Verification items for the finished model (mm, model axes). Face numbers are marked on the shaded views. A direction names the side the tool comes from. Round coordinates to 2 decimals unless told otherwise and drop trailing zeros. Order: outer loops, then holes, each group sorted by start corner. A loop starts at its lowest first (then second) coordinate and runs counter-clockwise, first axis right, second up. Notation, with made-up numbers: M 49.5,54.25 L 54.5,54.25 A19 cw 54.5,66.25 Z; hole C 43,69.25 d9. An arc over 180 degrees is marked long. Use CSV: the item, a comma, the result in double quotes. Start each with the question number.
Q1. Scan lines: line 1 (Z direction, x = 3.81, y = -4.7); line 2 (Y direction, x = 3, z = -6.5); line 3 (Y direction, x = 2.25, z = -15) (3 decimals). Record each from-to range of solid material in increasing order.
Q2. Sectioned sample at D-D (y = -91). Enter the section's corners in (x, z), and give its area (3 significant figures).
Q3. Sectioned sample at B-B (z = -4.5). Enter the section's corners in (x, y) (3 decimals).
Q4. Gauge pin test, flat ends, axial feed: pin 1 Ø4.5 at (x, y) = (8.26, -77.05) entering from -Z; pin 2 Ø1.7 at (x, y) = (9.5, -86) entering from +Z; pin 3 Ø4.5 at (x, z) = (3.81, -13.97) entering from -Y (3 decimals); pin 4 Ø3 at (x, z) = (3.81, -21.59) entering from -Y. Record the tip position at first contact, or that the pin passes through.
Q5. Sectioned sample at A-A (x = 3.81). Enter the section's corners in (y, z) (3 decimals), and give its area (3 significant figures).
Q6. Sectioned sample at C-C (z = -13.97). Enter the section's corners in (x, y) (3 decimals), and give its area (3 significant figures).
Q7. Set-up check for the marked faces 1, 2, 3 and 4: record each of +Z, -Z, +X, -X, +Y, -Y from which the full face is reachable in a straight line by a thin tool's end or side.
Q8. Mould release check, pull along Y, two halves, no side actions. Record for the marked faces 5, 6 and 7: +Y half, -Y half, draft (parallel to the pull), parting line (faces both ways), or undercut.
```python
from build123d import *

# Parameters (mm, degrees)
SKETCH1_W                                      = 12.7
SKETCH1_H                                      = 96.5962
EXTRUDE1_DEPTH                                 = 5.08
SKETCH2_W                                      = 12.7
SKETCH2_H                                      = 5.16498089
EXTRUDE2_DEPTH                                 = 25.4
F_4_CLEARANCE_HOLE1_D                          = 3.4544
SKETCH6_W                                      = 12.7
SKETCH6_H                                      = 22.86
EXTRUDE4_DEPTH                                 = 7.62
SKETCH7_W                                      = 7.9248
SKETCH7_H                                      = 15.24
EXTRUDE5_DEPTH                                 = 3.175
FILLET1_R                                      = 1.27
FILLET3_R                                      = 6.35
CHAMFER1_SIZE                                  = 0.762
CBORE_FOR_4_SOCKET_HEAD_CAP_SCREW1_D           = 3.4544
CBORE_FOR_4_SOCKET_HEAD_CAP_SCREW1_CBORE_D     = 5.55752
CBORE_FOR_4_SOCKET_HEAD_CAP_SCREW1_CBORE_DEPTH = 2.8448


with BuildPart() as part:
    # Sketch1 → Extrude1 (new body)
    with BuildSketch(Plane.XY):
        with Locations((6.35, -48.2981)):
            Rectangle(SKETCH1_W, SKETCH1_H)
    extrude(amount=EXTRUDE1_DEPTH)

    # Sketch2 → Extrude2 (add)
    with BuildSketch(Plane(origin=(0, 0, 0), x_dir=(-1, 0, 0), z_dir=(0, 0, -1))):
        with Locations((-6.35, -2.582490445)):
            Rectangle(SKETCH2_W, SKETCH2_H)
    extrude(amount=EXTRUDE2_DEPTH)

    # #4 Clearance Hole1 (through all)
    with Locations(Plane(origin=(0, 0, 0), x_dir=(-1, 0, 0), z_dir=(0, 1, 0))):
        with Locations((-3.81, -21.59), (-3.81, -13.97)):
            Hole(F_4_CLEARANCE_HOLE1_D / 2)

    # Sketch6 → Extrude4 (add)
    with BuildSketch(Plane(origin=(0, 0, 0), x_dir=(-1, 0, 0), z_dir=(0, 0, -1))):
        with Locations((-6.35, -85.1662)):
            Rectangle(SKETCH6_W, SKETCH6_H)
    extrude(amount=EXTRUDE4_DEPTH)

    # Sketch7 → Extrude5 (cut)
    with BuildSketch(Plane(origin=(0, 0, 0), x_dir=(1, 0, 0), z_dir=(0, 1, 0))):
        with Locations((3.81, 17.78)):
            Rectangle(SKETCH7_W, SKETCH7_H)
    extrude(amount=-EXTRUDE5_DEPTH, mode=Mode.SUBTRACT)

    # Fillet1
    fillet1_edges = [part.edges().sort_by_distance(p)[0] for p in [
        (7.7724, -1.5875, -10.16),
    ]]
    fillet(fillet1_edges, radius=FILLET1_R)

    # Fillet3
    fillet3_edges = [part.edges().sort_by_distance(p)[0] for p in [
        (6.35, -5.16498089, 0),
        (6.35, -73.7362, 0),
    ]]
    fillet(fillet3_edges, radius=FILLET3_R)

    # Chamfer1
    chamfer1_edges = [part.edges().sort_by_distance(p)[0] for p in [
        (12.7, -48.2981, 5.08),
        (6.35, 0, 5.08),
        (0, -48.2981, 5.08),
        (6.35, -96.5962, 5.08),
    ]]
    chamfer(chamfer1_edges, length=CHAMFER1_SIZE)

    # CBORE for #4 Socket Head Cap Screw1 (through all)
    with Locations(Plane.XY.offset(5.08)):
        with Locations((8.255, -84.97178089), (8.255, -77.04698089)):
            CounterBoreHole(CBORE_FOR_4_SOCKET_HEAD_CAP_SCREW1_D / 2, CBORE_FOR_4_SOCKET_HEAD_CAP_SCREW1_CBORE_D / 2, CBORE_FOR_4_SOCKET_HEAD_CAP_SCREW1_CBORE_DEPTH)


solid = part.part
```
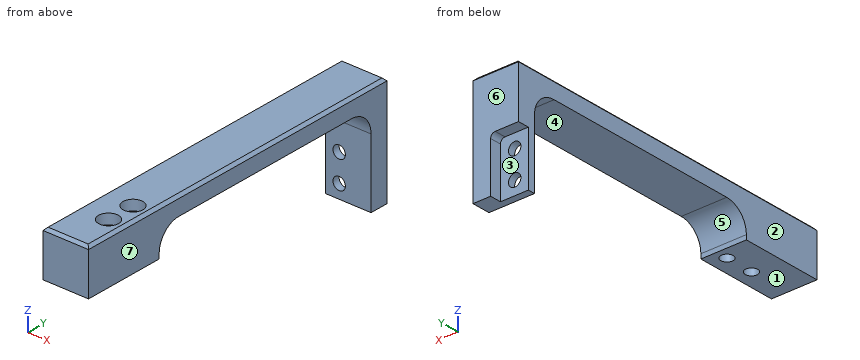
Verdict:
1,line 1,"z = -25.4 to -23.32, -19.86 to -15.7, -12.24 to 5.08"
1,line 2,"y = -96.6 to -73.74, -5.16 to 0"
1,line 3,"y = -5.165 to -3.175"
2,outline,"M 0,-7.62 L 12.7,-7.62 L 12.7,4.32 L 11.94,5.08 L 0.76,5.08 L 0,4.32 Z"
2,area,"161 mm²"
3,outline,"M 0,-96.596 L 12.7,-96.596 L 12.7,-73.461 L 0,-73.461 Z; M 0,-5.44 L 12.7,-5.44 L 12.7,0 L 0,0 Z; hole C 8.255,-84.972 d3.454; hole C 8.255,-77.047 d3.454"
4,pin 1,"stops at z = -7.62"
4,pin 2,"stops at z = 2.24"
4,pin 3,"stops at y = -5.165"
4,pin 4,"passes through"
5,outline,"M -96.596,-7.62 L -73.736,-7.62 L -73.736,-6.35 A6.35 cw -67.386,0 L -11.515,0 A6.35 cw -5.165,-6.35 L -5.165,-12.243 L -3.175,-12.243 L -3.175,-10.16 L 0,-10.16 L 0,4.318 L -0.762,5.08 L -95.834,5.08 L -96.596,4.318 Z; M -5.165,-25.4 L -3.175,-25.4 L -3.175,-23.317 L -5.165,-23.317 Z; M -5.165,-19.863 L -3.175,-19.863 L -3.175,-15.697 L -5.165,-15.697 Z"
5,area,"751 mm²"
6,outline,"M 0,-5.165 L 2.083,-5.165 L 2.083,-3.175 L 0,-3.175 Z; M 5.537,-5.165 L 12.7,-5.165 L 12.7,0 L 7.772,0 L 7.772,-3.175 L 5.537,-3.175 Z"
6,area,"34.0 mm²"
7,face 1,"-Z, +X, -X, -Y"
7,face 2,"+Z, -Z, -X, +Y, -Y"
7,face 3,"-Z, -X, +Y"
7,face 4,"-Z, +X, -X"
8,face 5,"undercut"
8,face 6,"+Y half"
8,face 7,"draft"
